Can you work these out from the model? Positions are in its coordinate system, mm. A direction names the side the tool comes from. Round coordinates to 2 decimals unless told otherwise and drop trailing zeros. Write each loop counter-clockwise with the first axis right and the second up, starting at its lowest first coordinate (ties: lowest second). Pieces come first, ordered by that corner, then holes. Notation, with made-up numbers: M -13,-5.5 L 9,-5.5 A29 ccw 9,31.5 Z; hole C -11,-18.5 d6. An arc over 180 degrees is marked long. Answer as a JSON object with one key per item and string values. Group by question number.
1) Please list where these lines run through material, in increasing order: L1, parallel to Z at x = -7.3, y = 0; L2, parallel to Z at x = -7.65, y = 0.5; L3, parallel to Y at x = -10.1, z = 0. Write a range as [from, to].
2) If we mould it in two halves opening along Z, with no side actions, what happens to faces 5 (the cylindrical face through (-6.48, 1.03, -38.35)), 6 (the cylindrical face through (-7, 0, 19)), 7 (the flat face through (-5, 0, -30)), 8 (the cylindrical face through (-6.5, 0.1, -40.5))? For each: +Z half, -Z half, draft (parallel to the pull), parting line (faces both ways), or undercut.
3) Suppose I cut it at A-A, the plane x = -6.7. Write out the boundary of the cut face in (y, z).
4) Suppose I cut it at D-D, the plane z = -11. Write out the boundary of the cut face in (x, y).
5) On a 3-axis mill with a long thin cutter (end or side, diameter ignored), from which of +Z, -Z, +X, -X, +Y, -Y can I reach the whole of each face in a straight line? I mean faces 1 (the cylindrical face through (-7, 0, -19)), 2 (the cylindrical face through (-9.52, 1.66, 0.37)), 3 (the cylindrical face through (-10, 0, 26)), 4 (the cylindrical face through (-10, 0, -26)). Say none if no direction works.
6) Suppose I cut it at C-C, the plane y = -1. Write out the boundary of the cut face in (x, z), and give its area (3 significant figures).
7) Suppose I cut it at B-B, the plane x = -9.75. Write out the boundary of the cut face in (y, z), and give its area (3 significant figures).
8) I'm going to push flat-ended pins straight in: pin 1 Ø2.5 at (y, z) = (0, 37) entering from -X (1 decimal); pin 2 Ø1 at (y, z) = (-1, -26.5) entering from -X; pin 3 Ø2 at (y, z) = (0, -10.5) entering from +X. Where does each tip first touch, or does it pass through?
Autodesk Inventor part; units mm, degrees
ref_plane "YZ Plane" through (0, 0, 0) normal (1, 0, 0) x (0, 1, 0)
ref_plane "XZ Plane" through (0, 0, 0) normal (0, 1, 0) x (-1, 0, 0)
ref_plane "XY Plane" through (0, 0, 0) normal (0, 0, 1) x (1, 0, 0)
sketch "Sketch1" plane through (0, 0, 0) normal (1, 0, 0) x (0, 1, 0)
  line L0 (0, -37) -> (0, 37) construction
  line L1 (3.5, -37) -> (3.5, 37)
  line L2 (-3.5, 37) -> (-3.5, -37)
  arc A0 (-3.5, -37) -> (3.5, -37) centre (0, -37) ccw
  arc A1 (3.5, 37) -> (-3.5, 37) centre (0, 37) ccw
  circle A2 centre (0, 37) radius 1.5
  circle A3 centre (0, 0) radius 1.5
  circle A4 centre (0, -37) radius 1.5
  line L3 (0, -22.5) -> (0, 22.5) construction
  line L4 (3.5, -22.5) -> (3.5, 22.5)
  line L5 (-3.5, 22.5) -> (-3.5, -22.5)
  arc A5 (-3.5, -22.5) -> (3.5, -22.5) centre (0, -22.5) ccw
  arc A6 (3.5, 22.5) -> (-3.5, 22.5) centre (0, 22.5) ccw
  line L6 (0, -37) -> (0, -22.5) construction
  line L7 (-3.5, -37) -> (-3.5, -22.5)
  line L8 (3.5, -22.5) -> (3.5, -37)
  arc A7 (-3.5, -37) -> (3.5, -37) centre (0, -37) ccw
  arc A8 (3.5, -22.5) -> (-3.5, -22.5) centre (0, -22.5) ccw
  line L9 (3.5, 0) -> (-3.5, 0) construction
  line L10 (0, 37) -> (0, 22.5) construction
  line L11 (-3.5, 37) -> (-3.5, 22.5)
  line L12 (3.5, 22.5) -> (3.5, 37)
  arc A9 (3.5, 37) -> (-3.5, 37) centre (0, 37) ccw
  arc A10 (-3.5, 22.5) -> (3.5, 22.5) centre (0, 22.5) ccw
  point P0 (0, -40.5)
  point P1 (0, 40.5)
  point P2 (0, -29.75)
  point P3 (0, 29.75)
  dimension "d18" = 81
  dimension "d19" = 3
  dimension "d20" = 7
  dimension "d32" = 45
extrude "Extrusión3" add sketch "Sketch1" along normal mid plane 22 contours A8 L2 A10 L1 | A5 A8 | A10 A6 | A3
extrude "Extrusión4" cut sketch "Sketch1" along normal mid plane 16 contours A8 L2 A10 L1 | A5 A8 | A10 A6 | A3
extrude "Extrusión5" add sketch "Sketch1" along normal mid plane 16 contours A0 L2 A5 L1 | A5 A8 | A6 L2 A1 L1 | A10 A6 | A2 | A4
extrude "Extrusión6" cut sketch "Sketch1" along normal mid plane 10 contours A0 L2 A5 L1 | A5 A8 | A6 L2 A1 L1 | A10 A6 | A2 | A4
sketch "Boceto2" plane through (-8, 0, 0) normal (-1, 0, 0) x (0, 0, 1)
  point P0 (-37, 0)
  point P1 (37, 0)
hole "Agujero1" at (-8, 0, -37) at (-8, 0, 37) direction (1, 0, 0) diameter 3.4 end through all
sketch "Boceto3" plane through (11, 0, 0) normal (1, 0, 0) x (0, 0, -1)
  point P0 (0, 0)
  point P1 (0, 0)
hole "Agujero2" at (11, 0, 0) direction (-1, 0, 0) diameter 3.4 end through all
sketch "Boceto4" plane through (11, 0, 0) normal (1, 0, 0) x (0, 0, -1)
  line L0 (-22.5, 3.5) -> (-37, 3.5)
  arc A0 (-37, 3.5) -> (-37, -3.5) centre (-37, 0) ccw
  line L1 (-37, -3.5) -> (-22.5, -3.5)
  line L2 (-22.5, -3.5) -> (22.5, -3.5)
  line L3 (22.5, 3.5) -> (-22.5, 3.5)
  line L4 (37, 3.5) -> (22.5, 3.5)
  arc A1 (37, -3.5) -> (37, 3.5) centre (37, 0) ccw
  line L5 (22.5, -3.5) -> (37, -3.5)
  point P0 (0, 0)
extrude "Extrusión7" cut sketch "Boceto4" against normal blind 10
equation "\"d35\" = Dedos"
equation "\"Dedos\" = 10"
properties part number "Corredera I"
Results:
{
 "1": {"L1": "[-40.5, -38.7], [-35.3, -19], [19, 35.3], [38.7, 40.5]", "L2": "[-40.46, -38.62], [-35.38, -19.04], [19.04, 35.38], [38.62, 40.46]", "L3": "[-3.5, -1.7], [1.7, 3.5]"},
 "2": {"face 5": "undercut", "face 6": "undercut", "face 7": "draft", "face 8": "-Z half"},
 "3": {"outline": "M -3.5,-37 A3.5 ccw 3.5,-37 L 3.5,-22.5 A3.5 ccw -3.5,-22.5 Z; M -3.5,22.5 A3.5 ccw 3.5,22.5 L 3.5,37 A3.5 ccw -3.5,37 Z; hole C 0,-37 d3.4; hole C 0,37 d3.4"},
 "4": {"outline": "M -11,-3.5 L -8,-3.5 L -8,3.5 L -11,3.5 Z"},
 "5": {"face 1": "+X", "face 2": "+X, -X", "face 3": "+Z, -X", "face 4": "-Z, -X"},
 "6": {"outline": "M -11,-25.85 L -8,-25.85 L -8,-35.63 L -5,-35.63 L -5,-19.15 L -8,-19.15 L -8,-1.37 L -11,-1.37 Z; M -11,1.37 L -8,1.37 L -8,19.15 L -5,19.15 L -5,35.63 L -8,35.63 L -8,25.85 L -11,25.85 Z; M -8,-40.35 L -5,-40.35 L -5,-38.37 L -8,-38.37 Z; M -8,38.37 L -5,38.37 L -5,40.35 L -8,40.35 Z", "area": "258 mm^2"},
 "7": {"outline": "M -3.5,-22.5 A3.5 ccw 3.5,-22.5 L 3.5,22.5 A3.5 ccw -3.5,22.5 Z; hole C 0,0 d3.4", "area": "344 mm^2"},
 "8": {"pin 1": "through", "pin 2": "x = -8", "pin 3": "x = -8"}
}
